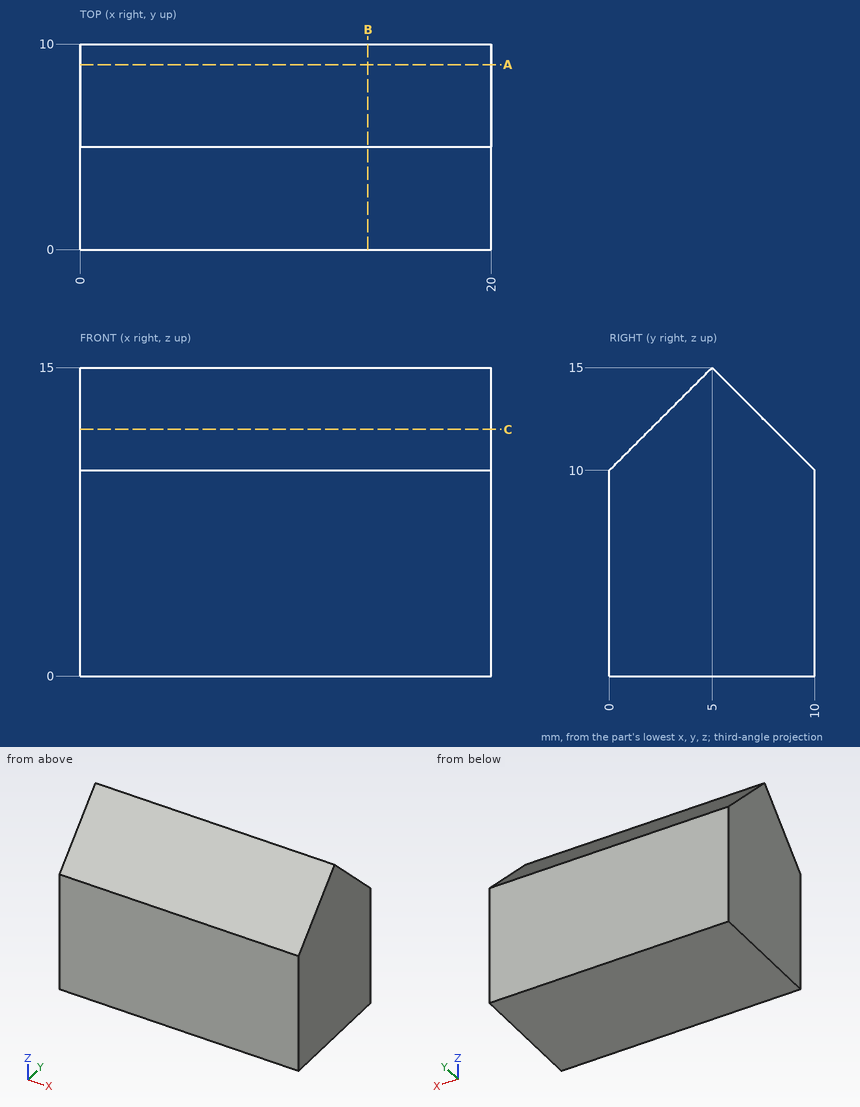
The figure shows three views and two pictorial views of one solid part (mm, origin at its lowest corner). Answer the questions. Give positions to 0.01 mm unless a question says otherwise; leave off trailing zeros. Order: outer loops, then holes, each group sorted by start corner. A loop starts at its lowest first (then second) coordinate and runs counter-clockwise, first axis right, second up. Notation, with made-up numbers: (-17, -1.75) -> (-2, -1.75) arc R20 cw to (-2, 12.25) -> close; hole circle Ø2 at (69, 71). An arc over 180 degrees is marked (long way). Answer as CSV lines item,"result". Start each with the question number.
(1) Section C-C, the plane z = 12 is taken. Write down the section's boundary in (x, y).
(2) Each of these flat-tipped pins is pushed along its axis until it touches: pin 1 Ø5 at (x, y) = (13, 7.5) entering from -Z; pin 2 Ø4 at (x, y) = (11.5, 7.5) entering from +Z. Where does it stop, or does it pass through?
(3) Section B-B, the plane x = 14 is taken. Write down the section's boundary in (y, z).
(4) Section A-A, the plane y = 9 is taken. Write down the section's boundary in (x, z), plus the area to 3 significant figures.
(5) Consider line 1 along Y through (x, z) = (15.5, 13.5); line 2 along Z through (x, y) = (12, 6.75); line 3 along Y through (x, z) = (16, 11.5). Determine where each line is inside the solid, lowest interval first.
Entries:
1,outline,"(0, 2) -> (20, 2) -> (20, 8) -> (0, 8) -> close"
2,pin 1,"z = 0"
2,pin 2,"z = 14.5"
3,outline,"(0, 0) -> (10, 0) -> (10, 10) -> (5, 15) -> (0, 10) -> close"
4,outline,"(0, 0) -> (20, 0) -> (20, 11) -> (0, 11) -> close"
4,area,"220 mm²"
5,line 1,"3.5 to 6.5"
5,line 2,"0 to 13.25"
5,line 3,"1.5 to 8.5"
